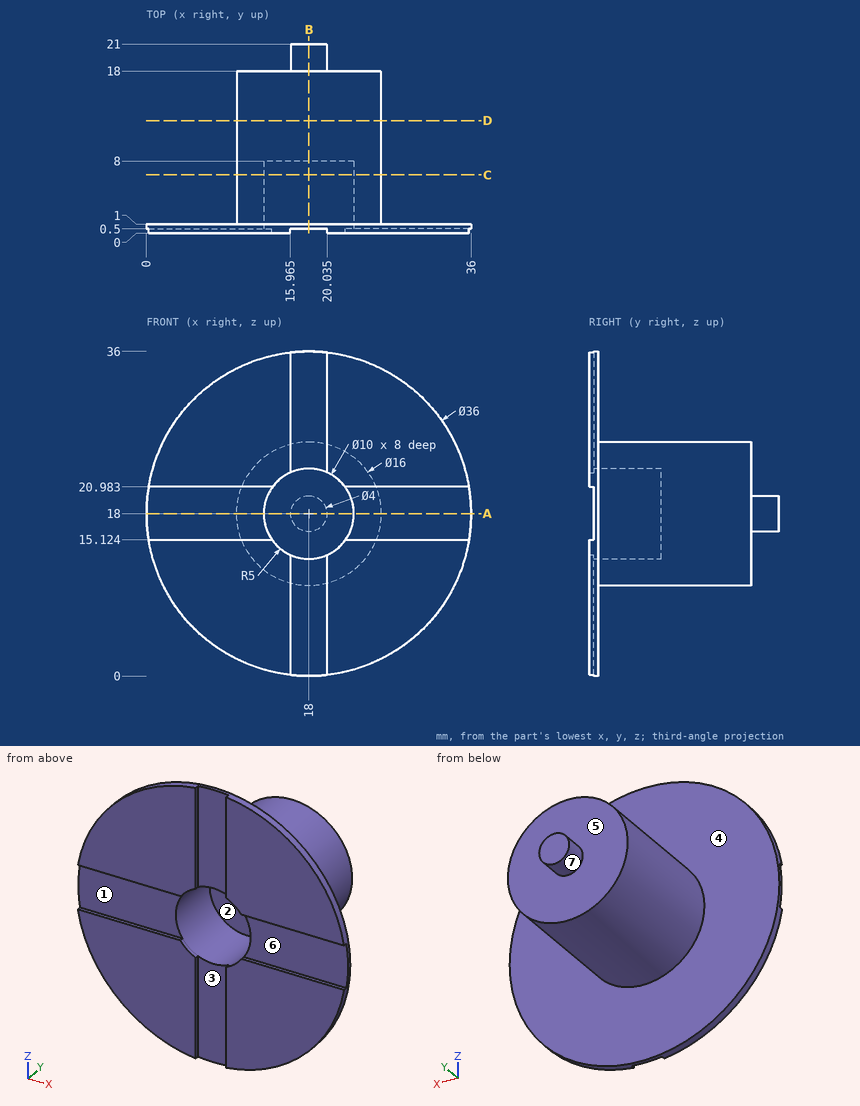
Verification items for this drawing (mm, ordinates from the low corner). A direction names the side the tool comes from. Coordinates: 2 decimals unless noted, no trailing zeros. Write each loop counter-clockwise with the first axis right and the second up, starting at its lowest first coordinate (ties: lowest second). Pieces come first, ordered by that corner, then holes. Notation, with made-up numbers: M 75.25,46 L 83.25,46 A6 ccw 83.25,52 Z; hole C 49.25,72.25 d10. An arc over 180 degrees is marked long. Answer as a JSON object with one key per item and string values. Group by question number.
(1) Gauge pin test, flat ends, axial feed: pin 1 (1.5 mm diameter, centred on x = 20.5, y = 19, fed in from -Z); pin 2 (8 mm diameter, centred on y = 4, z = 21.5, fed in from +X); pin 3 (5 mm diameter, centred on x = 5, z = 6, fed in from +Y). Record the tip position at first contact, or that the pin passes through.
(2) Release check for a two-part mould opening along Z. For the marked faces 5, 6 and 7 record: +Z half, -Z half, draft (parallel to the pull), parting line (faces both ways), or undercut.
(3) Cross-section at A-A, the plane z = 18. Record the cut outline in (x, y), and give its area (3 significant figures).
(4) Cross-section at B-B, the plane x = 18. Record the cut outline in (y, z), and give its area (3 significant figures).
(5) Cross-section at C-C, the plane y = 6.5. Record the cut outline in (x, z).
(6) Cross-section at D-D, the plane y = 12.5. Record the cut outline in (x, z), and give its area (3 significant figures).
(7) Material ranges on line 1 (X direction, y = 4.75, z = 18); line 2 (Y direction, x = 21.5, z = 24); line 3 (Y direction, x = 24.5, z = 11.5), recorded low to high.
(8) Tool access check on the marked faces 1, 2, 3 and 4. Record the directions out of +Z, -Z, +X, -X, +Y, -Y that give a thin tool (end or side, any length) a straight path to the whole face; none if there is none.
Reply:
{
 "1": {"pin 1": "z = 17.03", "pin 2": "x = 35.98", "pin 3": "y = 1"},
 "2": {"face 5": "draft", "face 6": "undercut", "face 7": "parting line"},
 "3": {"outline": "M 0,0.5 L 13,0.5 L 13,8 L 23,8 L 23,0.5 L 36,0.5 L 36,1 L 26,1 L 26,18 L 20,18 L 20,21 L 16,21 L 16,18 L 10,18 L 10,1 L 0,1 Z", "area": "227 mm²"},
 "4": {"outline": "M 0.5,0 L 1,0 L 1,10 L 18,10 L 18,16 L 21,16 L 21,20 L 18,20 L 18,26 L 1,26 L 1,36 L 0.5,36 L 0.5,23 L 8,23 L 8,13 L 0.5,13 Z", "area": "227 mm²"},
 "5": {"outline": "C 18,18 d16; hole C 18,18 d10"},
 "6": {"outline": "C 18,18 d16", "area": "201 mm²"},
 "7": {"line 1": "10 to 13, 23 to 26", "line 2": "0 to 18", "line 3": "0 to 1"},
 "8": {"face 1": "+X, -X, -Y", "face 2": "-Y", "face 3": "+Z, -Z, -Y", "face 4": "+Y"}
}
